Build history of the part. All positions in model axes, mm. A direction names the side the tool comes from. Give positions to 0.01 mm unless a question says otherwise; leave off trailing zeros. Write each loop counter-clockwise with the first axis right and the second up, starting at its lowest first coordinate (ties: lowest second). Pieces come first, ordered by that corner, then holes. Notation, with made-up numbers: (-29.5, 4.25) -> (-11.5, 4.25) arc R17 cw to (-11.5, 8.25) -> close; hole circle Ø5 at (6.25, 20). An arc over 180 degrees is marked (long way). Write item = value, one per line. Start each with the question number.
Q1. Saw through at A-A, the plane x = 57.15. List the corners of the cut face in (y, z) (3 decimals).
Q2. Tool access for faces 4 (the face through (54.85, 5.4, -17.48)), 5 (the face through (3.175, 13, -8)): list every direction of +Z, -Z, +X, -X, +Y, -Y with a clear straight run to the whole face (end or side of a thin tool).
Q3. Mould opens along X. For faces 1 (the face through (0, 13, -9)), 2 (the face through (34.237, 6.459, -17.485)), 3 (the face through (44, 13, -19.05)) say: pulls with the +X half, pulls with the -X half, needs draft (parallel to the pull), parting line crosses it, or undercut.
Q4. Saw through at D-D, the plane z = -12. List the corners of the cut face in (x, y) (3 decimals), then the cut area to 3 significant figures.
Q5. Saw through at C-C, the plane y = 6.35. List the corners of the cut face in (x, z) (3 decimals).
Q6. Saw through at B-B, the plane z = -6.35. List the corners of the cut face in (x, y) (3 decimals).
Q7. Wall check: line 1 (Y direction, x = 44.45, z = -17.2); line 2 (Y direction, x = 31.75, z = -16.8); line 3 (X direction, y = 1.25, z = -1.75) (3 decimals). Give the ranges that are in metal, low to high.
Q8. Drop flat-ended pins along their axis: P1, Ø3, axis at x = 31.75, y = 6.35, coming from the -Z side; P2, Ø6.5, axis at x = 44.45, y = 19.05, coming from the -Z side; P3, Ø5.5, axis at x = 44.45, y = 6.35, coming from the +Z side (3 decimals). Give the stop position or say it passes through.
from build123d import *

# Parameters (mm, degrees)
BOSS_EXTRUDE1_DEPTH     = 25.4
SKETCH2_R               = 3.175
CUT_EXTRUDE1_DEPTH      = 89.9
SKETCH3_R               = 3.175
CUT_EXTRUDE2_DEPTH      = 16.875
CUT_EXTRUDE2_DEPTH_BACK = 4.175
SKETCH4_R               = 2.4892
CUT_EXTRUDE3_DEPTH      = 4.175
SKETCH5_R               = 2.4892
CUT_EXTRUDE4_DEPTH      = 20.05


with BuildPart() as part:
    # Sketch1 → Boss-Extrude1 (new body)
    with BuildSketch(Plane(origin=(0, 0, 0), x_dir=(1, 0, 0), z_dir=(0, 1, 0))):
        Polygon((0, 0), (0, 19.05), (88.9, 19.05), (88.9, 0), (85.725, 0), (85.725, 15.875), (3.175, 15.875), (3.175, 0), align=None)
    extrude(amount=BOSS_EXTRUDE1_DEPTH)

    # Sketch2 → Cut-Extrude1 (cut, through all)
    with BuildSketch(Plane(origin=(88.9, 0, 0), x_dir=(0, 0, -1), z_dir=(1, 0, 0))):
        with Locations((6.35, 19.05)):
            Circle(SKETCH2_R)
    extrude(amount=-CUT_EXTRUDE1_DEPTH, mode=Mode.SUBTRACT)

    # Sketch3 → Cut-Extrude2 (cut, two sides)
    with BuildSketch(Plane.XY.offset(-15.875)) as cut_extrude2_sk:
        with Locations((12.7, 6.35)):
            Circle(SKETCH3_R)
        with Locations((76.2, 6.35)):
            Circle(SKETCH3_R)
    extrude(amount=CUT_EXTRUDE2_DEPTH, mode=Mode.SUBTRACT)
    extrude(cut_extrude2_sk.sketch, amount=-CUT_EXTRUDE2_DEPTH_BACK, mode=Mode.SUBTRACT)

    # Sketch4 → Cut-Extrude3 (cut, through all)
    with BuildSketch(Plane.XY.offset(-15.875)):
        with Locations((44.45, 19.05)):
            Circle(SKETCH4_R)
        with Locations((44.45, 6.35)):
            Circle(SKETCH4_R)
    extrude(amount=-CUT_EXTRUDE3_DEPTH, mode=Mode.SUBTRACT)

    # Sketch5 → Cut-Extrude4 (cut, through all)
    with BuildSketch(Plane(origin=(0, 0, -19.05), x_dir=(-1, 0, 0), z_dir=(0, 0, -1))):
        with Locations((-31.75, 6.35)):
            Circle(SKETCH5_R)
        with Locations((-57.15, 6.35)):
            Circle(SKETCH5_R)
    extrude(amount=-CUT_EXTRUDE4_DEPTH, mode=Mode.SUBTRACT)


solid = part.part
Report:
q1.outline = (0, -19.05) -> (3.861, -19.05) -> (3.861, -15.875) -> (0, -15.875) -> close; (8.839, -19.05) -> (25.4, -19.05) -> (25.4, -15.875) -> (8.839, -15.875) -> close
q2.face_4 = +Z, -Z
q2.face_5 = +Z, +Y, -Y
q3.face_1 = pulls with the -X half
q3.face_2 = undercut
q3.face_3 = needs draft
q4.outline = (0, 0) -> (3.175, 0) -> (3.175, 25.4) -> (0, 25.4) -> close; (85.725, 0) -> (88.9, 0) -> (88.9, 25.4) -> (85.725, 25.4) -> close
q4.area = 161 mm2
q5.outline = (0, -19.05) -> (9.525, -19.05) -> (9.525, -15.875) -> (3.175, -15.875) -> (3.175, 0) -> (0, 0) -> close; (15.875, -19.05) -> (29.261, -19.05) -> (29.261, -15.875) -> (15.875, -15.875) -> close; (34.239, -19.05) -> (41.961, -19.05) -> (41.961, -15.875) -> (34.239, -15.875) -> close; (46.939, -19.05) -> (54.661, -19.05) -> (54.661, -15.875) -> (46.939, -15.875) -> close; (59.639, -19.05) -> (73.025, -19.05) -> (73.025, -15.875) -> (59.639, -15.875) -> close; (79.375, -19.05) -> (88.9, -19.05) -> (88.9, 0) -> (85.725, 0) -> (85.725, -15.875) -> (79.375, -15.875) -> close
q6.outline = (0, 0) -> (3.175, 0) -> (3.175, 15.875) -> (0, 15.875) -> close; (0, 22.225) -> (3.175, 22.225) -> (3.175, 25.4) -> (0, 25.4) -> close; (85.725, 0) -> (88.9, 0) -> (88.9, 15.875) -> (85.725, 15.875) -> close; (85.725, 22.225) -> (88.9, 22.225) -> (88.9, 25.4) -> (85.725, 25.4) -> close
q7.line_1 = 0 to 3.86, 8.84 to 16.56, 21.54 to 25.4
q7.line_2 = 0 to 3.86, 8.84 to 25.4
q7.line_3 = 0 to 3.175, 85.725 to 88.9
q8.P1 = through
q8.P2 = -19.05
q8.P3 = -15.875
